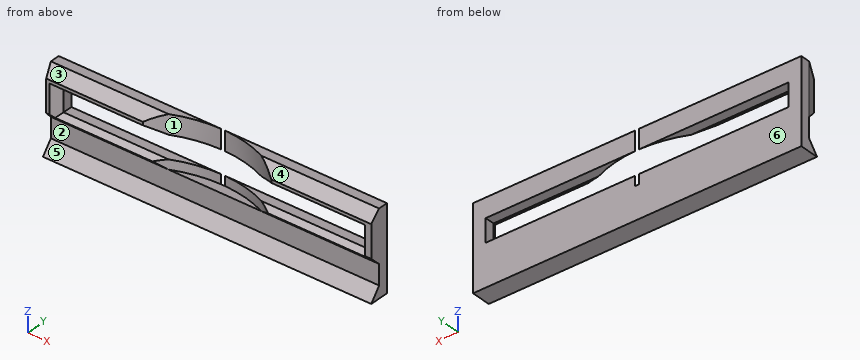
from build123d import *

# Parameters (mm, degrees)
PAD005_DEPTH       = 51
SKETCH018_W        = 11
SKETCH018_H        = 98
POCKET008_DEPTH    = 3
POCKET008_TAPER    = 33
SKETCH019_R        = 36.155756
POCKET009_DEPTH    = 16
CHAMFER003_SIZE2   = 1
CHAMFER003_SIZE    = 3
CHAMFER004_SIZE2   = 1
CHAMFER004_SIZE    = 3
POCKET008_FACE15_W = 94.103554
POCKET008_FACE15_H = 7.103554
POCKET010_DEPTH    = 5


with BuildPart() as part:
    # Sketch017 → Pad005 (new body, symmetric)
    with BuildSketch(Plane.YZ):
        Polygon((-74, 13), (-77, 13), (-80, 10), (-80, 8), (-80, 7.369175), (-80, 2.369175), (-80, 1), (-80, 0), (-77, -3), (-77, -9.20497), (-80, -13), (-74, -13), align=None)
    extrude(amount=PAD005_DEPTH, both=True)

    # Sketch018 (on Face10 of Pad005) → Pocket008 (cut)
    with BuildSketch(Plane(origin=(0, -80, 0), x_dir=(0, 0, -1), z_dir=(0, -1, 0))):
        with Locations((-3.5, 0)):
            Rectangle(SKETCH018_W, SKETCH018_H)
    extrude(amount=-POCKET008_DEPTH, taper=POCKET008_TAPER, mode=Mode.SUBTRACT)

    # Sketch019 (on Face9 of Pocket008) → Pocket009 (cut)
    with BuildSketch(Plane(origin=(0, 0, 13), x_dir=(0, -1, 0), z_dir=(0, 0, 1))):
        with Locations((110.149765, 0)):
            Circle(SKETCH019_R)
    extrude(amount=-POCKET009_DEPTH, mode=Mode.SUBTRACT)

    # Chamfer003
    chamfer003_edges = [part.edges().sort_by_distance(p)[0] for p in [
        (14.433704, -77, 3.5),
    ]]
    chamfer003_side = part.faces().sort_by_distance((10.734675, -75.624333, 5))[0]
    chamfer(chamfer003_edges, length=CHAMFER003_SIZE, length2=CHAMFER003_SIZE2, reference=chamfer003_side)

    # Chamfer004
    chamfer004_edges = [part.edges().sort_by_distance(p)[0] for p in [
        (-51, -80, 5),
    ]]
    chamfer004_side = part.faces().sort_by_distance((-51, -76.532918, 1.044872))[0]
    chamfer(chamfer004_edges, length=CHAMFER004_SIZE, length2=CHAMFER004_SIZE2, reference=chamfer004_side)

    # Pocket008 Face15 → Pocket010 (cut)
    with BuildSketch(Plane(origin=(0, -77, 3.5), x_dir=(-1, 0, 0), z_dir=(0, -1, 0))):
        Rectangle(POCKET008_FACE15_W, POCKET008_FACE15_H)
    extrude(amount=-POCKET010_DEPTH, mode=Mode.SUBTRACT)


solid = part.part
Can you work these out from the model? Positions are in its coordinate system, mm. Face numbers are marked on the shaded views. A direction names the side the tool comes from. Give positions to 0.01 mm unless a question says otherwise; leave off trailing zeros. Order: outer loops, then holes, each group sorted by start corner. A loop starts at its lowest first (then second) coordinate and runs counter-clockwise, first axis right, second up. Notation, with made-up numbers: M -28,76 L 17,76 A21 cw 17,80 Z; hole C -34,41 d4. An arc over 180 degrees is marked long. One line per item, written item: value.
Item 1: If we section it at C-C on x = -9: Write out the boundary of the cut face in (y, z).
Verdict:
outline: M -80,-13 L -74,-13 L -74,-0.05 L -75.13,-0.05 L -75.13,-3 L -77,-3 L -77,-9.2 Z; M -75.13,7.05 L -74,7.05 L -74,13 L -75.13,13 Z
Item 2: If we section it at A-A on x = 10.5: Write out the boundary of the cut face in (y, z).
Verdict:
outline: M -80,-13 L -74,-13 L -74,-0.05 L -75.55,-0.05 L -75.55,-3 L -77,-3 L -77,-9.2 Z; M -75.55,7.05 L -74,7.05 L -74,13 L -75.55,13 Z
Item 3: Please list where these lines run through material, in increasing order: line 1 (Z direction, x = -31.5, y = -74.5); line 2 (Z direction, x = 43, y = -77.25); line 3 (X direction, y = -79.5, z = 4.25).
Verdict:
line 1: -13 to -0.05, 7.05 to 13
line 2: -13 to -9.52, -2.75 to -0.21, 7.21 to 12.75
line 3: -50.17 to -48.68, 48.68 to 51
Item 4: If we mould it in two halves opening along Z, with no side actions, what happens to the marked faces 4, 5 and 6? For each: pulls with the +Z half, pulls with the -Z half, needs draft (parallel to the pull), parting line crosses it, or undercut.
Verdict:
face 4: pulls with the +Z half
face 5: undercut
face 6: needs draft
Item 5: If we section it at B-B on y = -76: Write out the boundary of the cut face in (x, z), and give its area (3 significant figures).
Verdict:
outline: M -51,-13 L 51,-13 L 51,13 L 11.88,13 L 11.88,7.05 L 47.05,7.05 L 47.05,-0.05 L 11.88,-0.05 L 11.88,-3 L -11.88,-3 L -11.88,-0.05 L -47.05,-0.05 L -47.05,7.05 L -11.88,7.05 L -11.88,13 L -51,13 Z
area: 1,770 mm2
Item 6: For the marked faces 1, 2 and 3, which set-ups out of +Z, -Z, +X, -X, +Y, -Y let a thin tool reach every point of the face, with its end or its side?
Verdict:
face 1: +Z, -Y
face 2: +X, -X, -Y
face 3: +Z, +X, -X, -Y
Item 7: For pin 1 (1 mm diameter, centred on x = -3, y = -77, fed in from +Z); pin 2 (5 mm diameter, centred on x = 14, z = -6, fed in from -Y); pin 3 (7 mm diameter, centred on x = -19, z = -5, fed in from -Y), each with a flat end and sliding along its axis, tell me the tip position at first contact or that it passes through.
Verdict:
pin 1: z = -3
pin 2: y = -77
pin 3: y = -78.5
